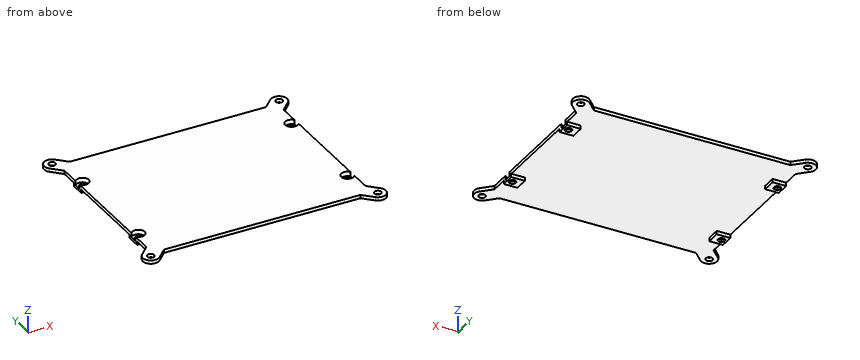
```python
from build123d import *

# Parameters (mm, degrees)
SKETCH_R        = 1.5
PAD_DEPTH       = 1.5
SKETCH001_W     = 6
SKETCH001_H     = 6
PAD001_DEPTH    = 1.5
SKETCH002_R     = 1.5
POCKET_DEPTH    = 3.001
SKETCH003_R     = 2.75
POCKET001_DEPTH = 2


with BuildPart() as part:
    # Sketch → Pad (new body)
    with BuildSketch(Plane.XY):
        with BuildLine():
            Line((-48.25, -33), (-48.25, 33))
            Line((-48.25, 33), (-52.492641, 37.242641))
            ThreePointArc((-47.492641, 42.242641), (-52.492641, 42.242641), (-52.492641, 37.242641))
            Line((-43.25, 38), (-47.492641, 42.242641))
            Line((-43.25, 38), (43.25, 38))
            Line((43.25, 38), (47.492641, 42.242641))
            ThreePointArc((52.492641, 37.242641), (52.492641, 42.242641), (47.492641, 42.242641))
            Line((48.25, 33), (52.492641, 37.242641))
            Line((48.25, 33), (48.25, -33))
            Line((48.25, -33), (52.492641, -37.242641))
            ThreePointArc((47.492641, -42.242641), (52.492641, -42.242641), (52.492641, -37.242641))
            Line((43.25, -38), (47.492641, -42.242641))
            Line((43.25, -38), (-43.25, -38))
            Line((-43.25, -38), (-47.492641, -42.242641))
            ThreePointArc((-52.492641, -37.242641), (-52.492641, -42.242641), (-47.492641, -42.242641))
            Line((-48.25, -33), (-52.492641, -37.242641))
        make_face()
        with Locations((49.992641, -39.742641)):
            Circle(SKETCH_R, mode=Mode.SUBTRACT)
        with Locations((-49.992641, -39.742641)):
            Circle(SKETCH_R, mode=Mode.SUBTRACT)
        with Locations((-49.992641, 39.742641)):
            Circle(SKETCH_R, mode=Mode.SUBTRACT)
        with Locations((49.992641, 39.742641)):
            Circle(SKETCH_R, mode=Mode.SUBTRACT)
    extrude(amount=PAD_DEPTH)

    # Sketch001 (on Face21 of Pad) → Pad001 (join)
    with BuildSketch(Plane(origin=(0, 0, 0), x_dir=(1, 0, 0), z_dir=(0, 0, -1))):
        with Locations((-45.25, 22.5)):
            Rectangle(SKETCH001_W, SKETCH001_H)
        with Locations((-45.25, -22.5)):
            Rectangle(SKETCH001_W, SKETCH001_H)
        with Locations((45.25, 22.5)):
            Rectangle(SKETCH001_W, SKETCH001_H)
        with Locations((45.25, -22.5)):
            Rectangle(SKETCH001_W, SKETCH001_H)
    extrude(amount=PAD001_DEPTH)

    # Sketch002 (on Face5 of Pad001) → Pocket (cut, through all)
    with BuildSketch(Plane.XY.offset(1.5)):
        with Locations((-46, 22.5)):
            Circle(SKETCH002_R)
        with Locations((-46, -22.5)):
            Circle(SKETCH002_R)
        with Locations((46, 22.5)):
            Circle(SKETCH002_R)
        with Locations((46, -22.5)):
            Circle(SKETCH002_R)
    extrude(amount=-POCKET_DEPTH, mode=Mode.SUBTRACT)

    # Sketch003 (on Face5 of Pocket) → Pocket001 (cut)
    with BuildSketch(Plane.XY.offset(1.5)):
        with Locations((46, 22.5)):
            Circle(SKETCH003_R)
        with Locations((-46, 22.5)):
            Circle(SKETCH003_R)
        with Locations((-46, -22.5)):
            Circle(SKETCH003_R)
        with Locations((46, -22.5)):
            Circle(SKETCH003_R)
    extrude(amount=-POCKET001_DEPTH, mode=Mode.SUBTRACT)


solid = part.part
```
Work out the finished part from the listing and answer in its coordinate system (mm). Give positions to 0.01 mm unless a question says otherwise; leave off trailing zeros. Loops run counter-clockwise (first coordinate to the right, second up) from the corner with the lowest first, then second, coordinate; pieces in that order, holes last. Notation, with made-up numbers: M 60,75 L 70,75 A24 ccw 70,109 Z; hole C 89,-17.5 d1. An arc over 180 degrees is marked long. One line per item, written item: value. Start each with the question number.
1. Find section C-C (y = -9). Give the vertices of the cut face in (x, z), and give its area (3 significant figures).
2. Find section B-B (y = 22.5). Give the vertices of the cut face in (x, z), and give its area (3 significant figures).
3. Each of these flat-tipped pins is pushed along its axis until it touches: P1, Ø3.5, axis at x = -46, y = -22.5, coming from the +Z side; P2, Ø4, axis at x = 28.5, y = 31.5, coming from the -Z side; P3, Ø2.5, axis at x = -46, y = -22.5, coming from the -Z side; P4, Ø0.8, axis at y = 21, z = -0.5, coming from the -X side. Where does it stop, or does it pass through?
4. Find section D-D (x = -10.5). Give the vertices of the cut face in (y, z).
5. Find the intervals of material crossed by probe 1 along Y at (x, z) = (-46, -0.9); probe 2 along Y at (x, z) = (-46, -0.05); probe 3 along X at (y, z) = (24.5, 0.6), in increasing order.
6. Find section A-A (x = -46). Give the vertices of the cut face in (y, z).
Reported:
1. outline: M -48.25,0 L 48.25,0 L 48.25,1.5 L -48.25,1.5 Z
1. area: 145 mm²
2. outline: M -48.25,-1.5 L -47.5,-1.5 L -47.5,-0.5 L -48.25,-0.5 Z; M -44.5,-1.5 L -42.25,-1.5 L -42.25,0 L 42.25,0 L 42.25,-1.5 L 44.5,-1.5 L 44.5,-0.5 L 43.25,-0.5 L 43.25,1.5 L -43.25,1.5 L -43.25,-0.5 L -44.5,-0.5 Z; M 47.5,-1.5 L 48.25,-1.5 L 48.25,-0.5 L 47.5,-0.5 Z
2. area: 137 mm²
3. P1: stops at z = -0.5
3. P2: stops at z = 0
3. P3: passes through
3. P4: stops at x = -48.25
4. outline: M -38,0 L 38,0 L 38,1.5 L -38,1.5 Z
5. probe 1: y = -25.5 to -24, -21 to -19.5, 19.5 to 21, 24 to 25.5
5. probe 2: y = -25.5 to -25.25, -19.75 to -19.5, 19.5 to 19.75, 25.25 to 25.5
5. probe 3: x = -48.25 to -47.89, -44.11 to 44.11, 47.89 to 48.25
6. outline: M -40.75,0 L -25.5,0 L -25.5,-1.5 L -24,-1.5 L -24,-0.5 L -25.25,-0.5 L -25.25,1.5 L -40.75,1.5 Z; M -21,-1.5 L -19.5,-1.5 L -19.5,0 L 19.5,0 L 19.5,-1.5 L 21,-1.5 L 21,-0.5 L 19.75,-0.5 L 19.75,1.5 L -19.75,1.5 L -19.75,-0.5 L -21,-0.5 Z; M 24,-1.5 L 25.5,-1.5 L 25.5,0 L 40.75,0 L 40.75,1.5 L 25.25,1.5 L 25.25,-0.5 L 24,-0.5 Z
